Autodesk Fusion 360 part; units mm, degrees
sketch "Plate" plane through (0, 0, 0) normal (0, 1, 0) x (1, 0, 0)
  line L0 (0, 0) -> (5, 0)
  line L1 (5, 0) -> (5, -90)
  line L2 (5, -90) -> (0, -90)
  line L3 (0, -90) -> (0, 0)
  dimension "d67" = 5
  dimension "d68" = 90
extrude "Plate (1)" add sketch "Plate" along normal mid plane 24
sketch "Hook profile" plane through (0, 0, 0) normal (0, 1, 0) x (1, 0, 0)
  line L0 (0, -88) -> (-8.3, -88)
  line L1 (-8.3, -88) -> (-8.3, -71)
  line L2 (-8.3, -71) -> (-5.3, -71)
  line L3 (-5.3, -71) -> (-3.8, -72.5)
  line L4 (-3.8, -72.5) -> (-3.8, -83)
  line L5 (-3.8, -83) -> (0, -83)
  line L6 (0, -83) -> (0, -88)
  dimension "d71" = 88
  dimension "d72" = 8.3
  dimension "d73" = 3.8
  dimension "d74" = 5
  dimension "d75" = 10.5
  dimension "d76" = 1.5
  dimension "d77" = 1.5
extrude "Hook profile (1)" add sketch "Hook profile" along normal mid plane 2.4
pattern_linear "Hook rows" count 4 spacing 25.4 along (0, 0, -1) count 3 spacing 0 along (0, 0, 1) of "Hook profile (1)"
equation "bracketWidth = 24.0 mm"
equation "hookTabWidth = slotWidth - 0.8 mm"
equation "slotPitchVertical = 25.4 mm"
equation "slotWidth = 3.2 mm"
equation "faceMetalThickness = 2.0 mm"
equation "hookThroat = faceMetalThickness + 1.8 mm"
equation "hookNeckHeight = 5.0 mm"
equation "hookLipThickness = 4.5 mm"
equation "hookLipDrop = 12.0 mm"
equation "plateHeight = 90.0 mm"
equation "gaugePlateThickness = 5.0 mm"
equation "hookLipChamfer = 1.5 mm"
equation "topHookNeckTop = 88.0 mm"
equation "d67 = gaugePlateThickness"
equation "d68 = plateHeight"
equation "d69 = bracketWidth"
equation "d71 = topHookNeckTop"
equation "d72 = hookThroat + hookLipThickness"
equation "d73 = hookThroat"
equation "d74 = hookNeckHeight"
equation "d75 = hookLipDrop - hookLipChamfer"
equation "d76 = hookLipChamfer"
equation "d77 = hookLipChamfer"
equation "d78 = hookTabWidth"
Model file for the job. Use its own axes, mm. A direction names the side the tool comes from. Round coordinates to 2 decimals unless told otherwise and drop trailing zeros. Write each loop counter-clockwise with the first axis right and the second up, starting at its lowest first coordinate (ties: lowest second). Pieces come first, ordered by that corner, then holes. Notation, with made-up numbers: (-32, 48) -> (8, 48) arc R12 ccw to (8, 68) -> close; hole circle Ø4 at (22.25, 77). An arc over 180 degrees is marked (long way). Answer as CSV lines item,"result".
1. Tool access for faces 1 (the face through (-3.8, 0, 78)), 2 (the face through (-7, 0, 71)), 3 (the face through (-5, -1.2, 30)), 4 (the face through (-3.8, 0, 1)): list every direction of +Z, -Z, +X, -X, +Y, -Y with a clear straight run to the whole face (end or side of a thin tool).
Resolved:
face 1,"+Y, -Y"
face 2,"-X, +Y, -Y"
face 3,"+Z, -Z, -X, -Y"
face 4,"-Z, +Y, -Y"
2. Pin check, flat tips, straight feed: pin 1 Ø1.9 at (x, y) = (-6, 0) entering from +Z; pin 2 Ø12 at (y, z) = (-1.5, 7.5) entering from -X; pin 3 Ø0.7 at (x, y) = (-2.5, 0.5) entering from -Z; pin 4 Ø2.5 at (x, z) = (-5, 5) entering from +Y. Stop position of each tip, or through.
Resolved:
pin 1,"z = 88"
pin 2,"x = -8.3"
pin 3,"z = 6.8"
pin 4,"y = 1.2"
3. Slice it at B-B, the plane x = -7.5. List the corners of the cut face in (y, z).
Resolved:
outline,"(-1.2, -5.2) -> (1.2, -5.2) -> (1.2, 11.8) -> (-1.2, 11.8) -> close; (-1.2, 20.2) -> (1.2, 20.2) -> (1.2, 37.2) -> (-1.2, 37.2) -> close; (-1.2, 45.6) -> (1.2, 45.6) -> (1.2, 62.6) -> (-1.2, 62.6) -> close; (-1.2, 71) -> (1.2, 71) -> (1.2, 88) -> (-1.2, 88) -> close"
4. Mould opens along X. For faces 5 (the face through (-8.3, 0, 80)), 6 (the face through (-5, -1.2, 81)), 7 (the face through (-3.8, 0, 52)) say: +X half, -X half, draft (parallel to the pull), parting line (faces both ways), or undercut.
Resolved:
face 5,"-X half"
face 6,"draft"
face 7,"undercut"
5. Drill centre lines: line 1 (Z direction, x = -7, y = -1); line 2 (Y direction, x = -5.5, z = 23.5); line 3 (X direction, y = 0.25, z = 15). Where is each one in solid material? Low to high.
Resolved:
line 1,"-5.2 to 11.8, 20.2 to 37.2, 45.6 to 62.6, 71 to 88"
line 2,"-1.2 to 1.2"
line 3,"0 to 5"
6. Slice it at D-D, the plane z = 35.5. List the corners of the cut face in (x, y), plus the area to 3 significant figures.
Resolved:
outline,"(-8.3, -1.2) -> (0, -1.2) -> (0, -12) -> (5, -12) -> (5, 12) -> (0, 12) -> (0, 1.2) -> (-8.3, 1.2) -> close"
area,"140 mm²"
7. Slice it at A-A, the plane z = 5. List the corners of the cut face in (x, y), plus the area to 3 significant figures.
Resolved:
outline,"(-8.3, -1.2) -> (-3.8, -1.2) -> (-3.8, 1.2) -> (-8.3, 1.2) -> close; (0, -12) -> (5, -12) -> (5, 12) -> (0, 12) -> close"
area,"131 mm²"
